Verification items for the finished model (mm, model axes). Face numbers are marked on the shaded views. A direction names the side the tool comes from. Coordinates: 2 decimals unless noted, no trailing zeros. Write each loop counter-clockwise with the first axis right and the second up, starting at its lowest first coordinate (ties: lowest second). Pieces come first, ordered by that corner, then holes. Notation, with made-up numbers: M -39,-1.5 L -32,-1.5 A13 ccw -32,10.5 Z; hole C 82,31.5 d2. An arc over 180 degrees is marked long. One line per item, written item: value.
Autodesk Inventor part; units mm, degrees
ref_plane "YZ Plane" through (0, 0, 0) normal (1, 0, 0) x (0, 1, 0)
ref_plane "XZ Plane" through (0, 0, 0) normal (0, 1, 0) x (-1, 0, 0)
ref_plane "XY Plane" through (0, 0, 0) normal (0, 0, 1) x (1, 0, 0)
sketch "Sketch1" plane through (0, 0, 0) normal (0, 0, 1) x (1, 0, 0)
  arc A0 (-18, 0) -> (18, 0) centre (0, 0) ccw
  line L0 (-18, 0) -> (-18, 35)
  line L1 (18, 0) -> (18, 35)
  line L2 (-18, 35) -> (18, 35)
  dimension "d0" = 36
  dimension "d2" = 35
extrude "Extrusion1" add sketch "Sketch1" against normal mid plane 15
sketch "Sketch2" plane through (0, 0, 0) normal (1, 0, 0) x (0, 1, 0)
  line L0 (35, -7.5) -> (0, -7.5)
  line L1 (35, -7.5) -> (35, 7.5)
  arc A0 (42.5, -15) -> (35, -7.5) centre (35, -15) ccw
  line L2 (42.5, -47.5) -> (42.5, -15)
  line L3 (42.5, -47.5) -> (67.5, -47.5)
  line L4 (67.5, -47.5) -> (67.5, -7.5)
  line L5 (60, 0) -> (35, 0)
  arc A1 (67.5, -7.5) -> (60, 0) centre (60, -7.5) ccw
  point P0 (0, 0)
  dimension "d10" = 40
  dimension "d11" = 25
  dimension "d12" = 15
extrude "Extrusion2" add sketch "Sketch2" along normal mid plane 36
sketch "Sketch3" plane through (0, 0, 0) normal (1, 0, 0) x (0, 1, 0)
  line L0 (42.5, -47.5) -> (67.5, -47.5)
  line L1 (-18, -7.5) -> (0, -7.5)
  line L2 (42.5, -47.5) -> (-18, -7.5)
  line L3 (35, -7.5) -> (0, -7.5)
  arc A0 (42.5, -15) -> (35, -7.5) centre (35, -15) ccw
  line L4 (42.5, -15) -> (42.5, -47.5)
  point P0 (0, 0)
extrude "Extrusion3" add sketch "Sketch3" along normal mid plane 15
delete faces "Delete Face1" heal yes whole lump no faces at (-6.6957, -17.2098, -7.5) (6.6957, -17.2098, -7.5)
fillet "Fillet1" radius 2 6 edges at (-7.5, 40.3033, -9.6967) (-7.5, 42.5, -31.25) (-7.5, 9.3185, -7.5) (7.5, 42.5, -31.25) (7.5, 9.3185, -7.5) (7.5, 40.3033, -9.6967)
sketch "Sketch5" plane through (0, 0, 0) normal (1, 0, 0) x (0, 1, 0)
  line L0 (47.5, -54.8971) -> (47.5, 0)
  line L1 (67.5, -47.5) -> (67.5, -7.5)
  line L2 (0, -7.5) -> (0, 7.5)
  line L3 (35, -7.5) -> (0, -7.5)
  arc A0 (42.5, -15) -> (35, -7.5) centre (35, -15) ccw
  line L4 (42.5, -15) -> (42.5, -47.5)
  line L5 (42.5, -47.5) -> (67.5, -47.5)
  line L6 (67.5, -47.5) -> (67.5, -7.5)
  arc A1 (67.5, -7.5) -> (60, 0) centre (60, -7.5) ccw
  line L7 (60, 0) -> (35, 0)
  line L8 (35, 0) -> (35, 7.5)
  line L9 (0, 7.5) -> (35, 7.5)
  point P0 (0, 0)
  point P1 (47.5, -47.5)
  dimension "d21" = 20
extrude "Extrusion5" cut sketch "Sketch5" against normal mid plane 24 contours L0 L7 A1 L1 L5
sketch "Sketch6" plane through (0, 0, 7.5) normal (0, 0, 1) x (1, 0, 0)
  arc A0 (-18, 0) -> (18, 0) centre (0, 0) ccw
  line L0 (18, 0) -> (18, 35)
  line L1 (18, 35) -> (-18, 35)
  line L2 (-18, 35) -> (-18, 0)
  arc A1 (-16.5, 0) -> (16.5, 0) centre (0, 0) ccw
  line L3 (-16.5, 0) -> (-16.5, 33.5)
  line L4 (-16.5, 33.5) -> (16.5, 33.5)
  line L5 (16.5, 33.5) -> (16.5, 0)
  dimension "d24" = 1.5
extrude "Extrusion6" cut sketch "Sketch6" against normal blind 0.25 contours L3 L4 L5 A1
fillet "Fillet2" radius 5 2 edges at (-18, 55, -47.5) (18, 55, -47.5)
sketch "Sketch7" plane through (-18, 35, 0) normal (-1, 0, 0) x (0, 0, 1)
  line L0 (-42.5, 7.5) -> (-42.5, 32.5)
  line L1 (-42.5, 7.5) -> (-15, 7.5)
  arc A0 (-7.5, 0) -> (-15, 7.5) centre (-15, 0) ccw
  line L2 (-7.5, -35) -> (-7.5, 0)
  line L3 (7.5, -35) -> (-7.5, -35)
  line L4 (7.5, 0) -> (7.5, -35)
  line L5 (0, 0) -> (7.5, 0)
  line L6 (0, 0) -> (0, 25)
  arc A1 (0, 25) -> (-7.5, 32.5) centre (-7.5, 25) ccw
  line L7 (-7.5, 32.5) -> (-42.5, 32.5)
  circle A2 centre (-12.5, 20) radius 6
  line L8 (-47.5, 32.5) -> (-47.5, 7.5)
  circle A3 centre (-35, 20) radius 6
  point P0 (0, -35)
  point P1 (-47.5, 20)
  dimension "d28" = 25
  dimension "d29" = 12
  dimension "d30" = 47.5
  dimension "d31" = 12.5
  dimension "d32" = 12
  dimension "d33" = 12.5
extrude "Extrusion7" cut sketch "Sketch7" against normal through all contours A2 | A3
properties part number "Holder of gripper"
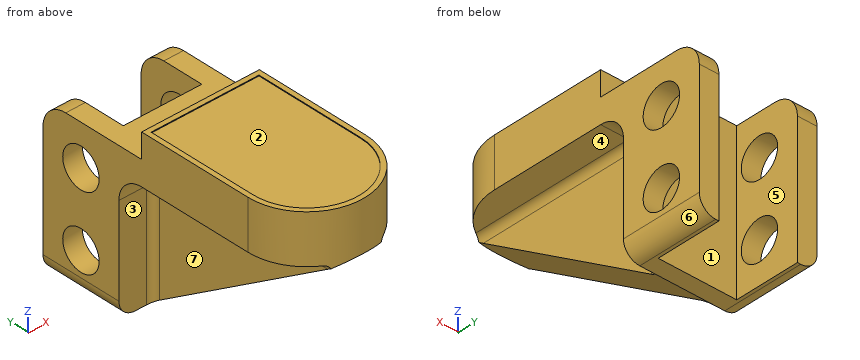
Item 1: Cross-section at A-A, the plane z = -35. Enter the section's corners in (x, y), and give its area (3 significant figures).
The answers:
outline: M -18,42.5 L -9.5,42.5 A2 cw -7.5,40.5 L -7.5,23.59 L 7.5,23.59 L 7.5,40.5 A2 cw 9.5,42.5 L 18,42.5 L 18,49 L 12,49 L 12,47.5 L -12,47.5 L -12,49 L -18,49 Z; M -18,61 L -12,61 L -12,67.5 L -18,67.5 Z; M 12,61 L 18,61 L 18,67.5 L 12,67.5 Z
area: 561 mm²
Item 2: Go/stop test with flat-tipped pins: P1, Ø6, axis at x = 7, y = 13, coming from the -Z side; P2, Ø4, axis at x = -6.5, z = -3, coming from the +Y side; P3, Ø7.5, axis at x = 1.5, y = 47, coming from the +Z side. Record where each tip stops, or that it passes through.
The answers:
P1: stops at z = -29.98
P2: stops at y = 47.5
P3: stops at z = 0
Item 3: Cross-section at D-D, the plane z = -4.5. Enter the section's corners in (x, y), and give its area (3 significant figures).
The answers:
outline: M -18,0 A18 ccw 18,0 L 18,66.87 L 12,66.87 L 12,47.5 L -12,47.5 L -12,66.87 L -18,66.87 Z
area: 2,450 mm²
Item 4: Cross-section at B-B, the plane x = 0. Enter the section's corners in (y, z).
The answers:
outline: M -18,-7.5 L 42.5,-47.5 L 47.5,-47.5 L 47.5,0 L 35,0 L 35,7.5 L 33.5,7.5 L 33.5,7.25 L -16.5,7.25 L -16.5,7.5 L -18,7.5 Z
Item 5: Draft check along X on the marked faces 5, 6 and 7. Enter one of: released by +X, released by -X, zero draft, split by the parting line, or undercut.
The answers:
face 5: undercut
face 6: released by +X
face 7: released by -X
Item 6: Cross-section at C-C, the plane y = 10. Enter the section's corners in (x, z), and give its area (3 significant figures).
The answers:
outline: M -18,-7.5 L -9.5,-7.5 A2 cw -7.5,-9.5 L -7.5,-26.01 L 7.5,-26.01 L 7.5,-9.5 A2 cw 9.5,-7.5 L 18,-7.5 L 18,7.5 L 16.5,7.5 L 16.5,7.25 L -16.5,7.25 L -16.5,7.5 L -18,7.5 Z
area: 811 mm²
Item 7: Scan lines: line 1 (Y direction, x = -13.7, z = -35); line 2 (X direction, y = 27, z = -13.5); line 3 (Z direction, x = 11, y = -8). Record each from-to range of solid material in increasing order.
The answers:
line 1: y = 42.5 to 49, 61 to 67.5
line 2: x = -7.5 to 7.5
line 3: z = -7.5 to 7.25
Item 8: Access from +Z, -Z, +X, -X, +Y, -Y to the whole of each face (thin tool, end or side, straight path). Record for the marked faces 1, 2, 3 and 4.
The answers:
face 1: +Z, -Z, +Y
face 2: +Z
face 3: -Z, -X, -Y
face 4: -Z, +X, -Y
